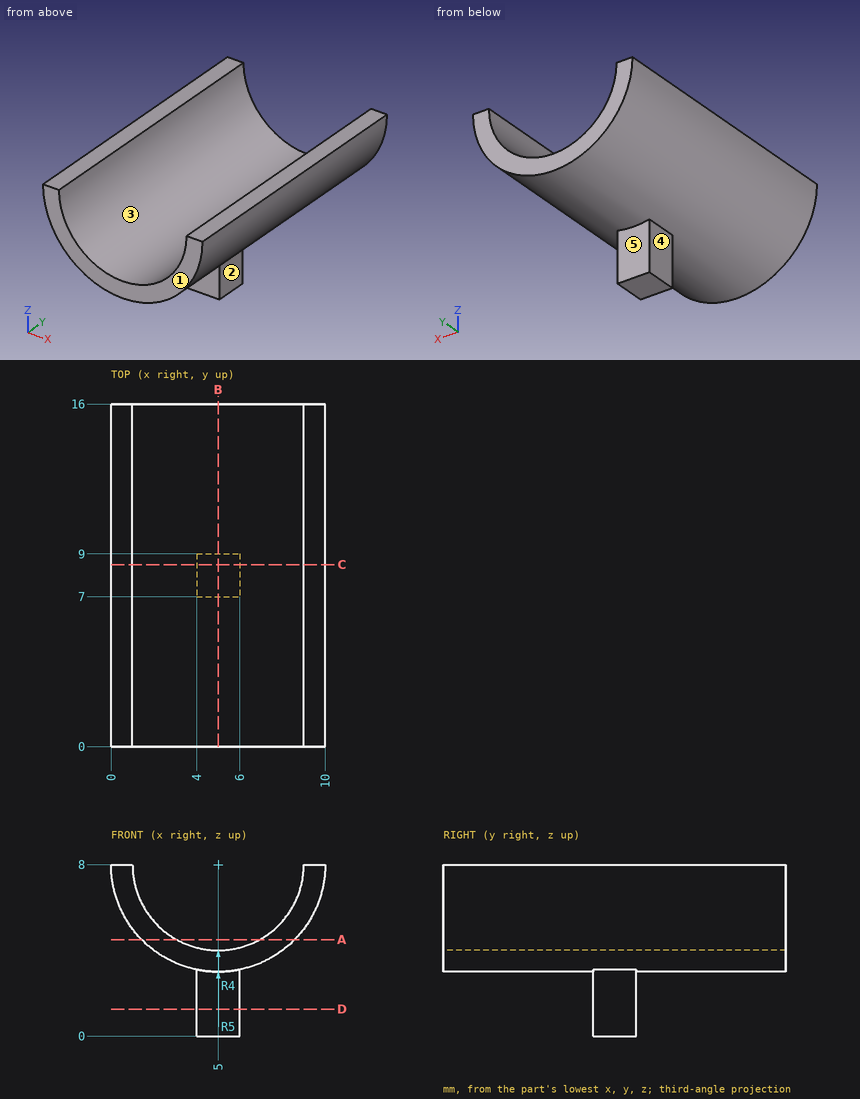
Source: three-view drawing plus pictorial views. Frame: mm from the lowest corner of the part. A direction names the side the tool comes from. Round coordinates to 2 decimals unless told otherwise and drop trailing zeros. Order: outer loops, then holes, each group sorted by start corner. A loop starts at its lowest first (then second) coordinate and runs counter-clockwise, first axis right, second up. Notation, with made-up numbers: (16, 71) -> (45, 71) arc R22 ccw to (45, 109) -> close; hole circle Ø1 at (-13, 23.5). An arc over 180 degrees is marked (long way). Use one line per item in the form item = value. Start each with the question number.
1. Cut plane C-C (y = 8.5). Return the cut outline in (x, z), then the cut area to 3 significant figures.
2. Cut plane B-B (x = 5). Return the cut outline in (y, z), then the cut area to 3 significant figures.
3. Cut plane D-D (z = 1.25). Return the cut outline in (x, y).
4. Reachability of the marked faces 1 and 2 from +Z, -Z, +X, -X, +Y, -Y: full face, straight path, thin tool, end or side. Return the list, or none.
5. Pin query (flat end, axial travel): pin 1 Ø0.6 at (y, z) = (8.5, 1.5) entering from +X; pin 2 Ø2 at (y, z) = (14, 2.5) entering from +X; pin 3 Ø1.6 at (x, z) = (5, 2) entering from -Y. Return the tip coordinate at first contact, or that it passes through.
6. Line query: probe 1 along X at (y, z) = (12, 6.5); probe 2 along X at (y, z) = (3.5, 7.5); probe 3 along Z at (x, y) = (0.5, 13.5). Output: solid intervals per line, ascending.
7. Cut plane A-A (z = 4.5). Return the cut outline in (x, y).
8. Draft query along X for the marked faces 3, 4 and 5. Return one class per face: pulls with the +X half, pulls with the -X half, needs draft (parallel to the pull), parting line crosses it, or undercut.
Solution:
q1.outline = (0, 8) arc R5 ccw to (4, 3.1) -> (4, 0) -> (6, 0) -> (6, 3.1) arc R5 ccw to (10, 8) -> (9, 8) arc R4 cw to (1, 8) -> close
q1.area = 20.2 mm^2
q2.outline = (0, 3) -> (7, 3) -> (7, 0) -> (9, 0) -> (9, 3) -> (16, 3) -> (16, 4) -> (0, 4) -> close
q2.area = 22.0 mm^2
q3.outline = (4, 7) -> (6, 7) -> (6, 9) -> (4, 9) -> close
q4.face_1 = +Z, -Z, +X, -X, -Y
q4.face_2 = -Z, +X, +Y, -Y
q5.pin_1 = 6
q5.pin_2 = 7.18
q5.pin_3 = 7
q6.probe_1 = 0.23 to 1.29, 8.71 to 9.77
q6.probe_2 = 0.03 to 1.03, 8.97 to 9.97
q6.probe_3 = 5.82 to 8
q7.outline = (1.43, 0) -> (3.06, 0) -> (3.06, 16) -> (1.43, 16) -> close; (6.94, 0) -> (8.57, 0) -> (8.57, 16) -> (6.94, 16) -> close
q8.face_3 = undercut
q8.face_4 = pulls with the -X half
q8.face_5 = needs draft
